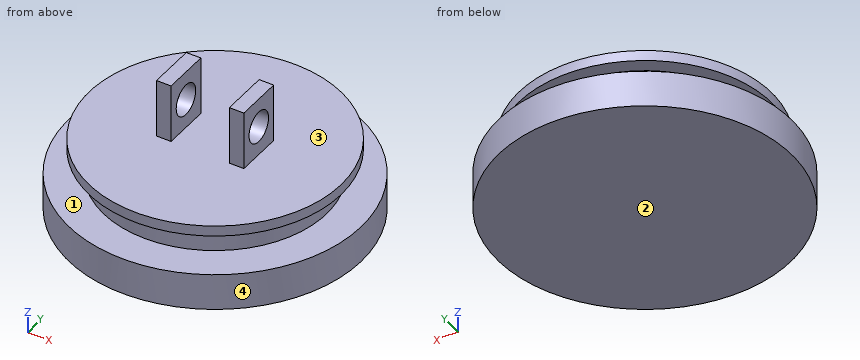
from build123d import *

# Parameters (mm, degrees)
F0_R      = 20
F1_DEPTH  = 5
F2_R      = 17.25
F3_DEPTH  = 10
F4_W      = 2
F4_H      = 3.56
F7_W      = 2
F7_H      = 6.5
F8_DEPTH  = 8
F9_R      = 2.125
F10_DEPTH = 26.001


with BuildPart() as f1:
    # F0 (on Top) → F1 (new body)
    with BuildSketch(Plane.XY):
        Circle(F0_R)
    extrude(amount=F1_DEPTH)

    # F2 (on Top) → F3 (join)
    with BuildSketch(Plane.XY):
        Circle(F2_R)
    extrude(amount=F3_DEPTH)

    # F4 (on Right) → F6 (revolve, cut)
    with BuildSketch(Plane.YZ):
        with Locations((16.25, 6.78)):
            Rectangle(F4_W, F4_H)
    revolve(axis=Axis((0, 0, 6.819869), (0, 0, 1)), mode=Mode.SUBTRACT)

    # F7 (on face) → F8 (join)
    with BuildSketch(Plane.XY.offset(10)):
        with Locations((5, 0)):
            Rectangle(F7_W, F7_H)
        with Locations((-5, 0)):
            Rectangle(F7_W, F7_H)
    extrude(amount=F8_DEPTH)

    # F9 (on face) → F10 (cut, through all)
    with BuildSketch(Plane(origin=(-6, 0, 0), x_dir=(0, -1, 0), z_dir=(-1, 0, 0))):
        with Locations((0, 14)):
            Circle(F9_R)
    extrude(amount=-F10_DEPTH, mode=Mode.SUBTRACT)


solid = f1.part
Design review of the part built by this model. Coordinates are the model's own, in mm. Face numbers are marked on the shaded views. Round coordinates to 2 decimals unless told otherwise and drop trailing zeros. Loops run counter-clockwise (first coordinate to the right, second up) from the corner with the lowest first, then second, coordinate; pieces in that order, holes last. Notation, with made-up numbers: M -29,66 L 6,66 A14 ccw 6,81 Z; hole C 25,16.5 d6. An arc over 180 degrees is marked long. Answer as a JSON object with one key per item and string values.
Item 1: We need section A-A on y = 0. Give the boundary of the cut face in (x, z) (3 decimals), and give its area (3 significant figures).
Answer sheet:
{"outline": "M -20,0 L 20,0 L 20,5 L 15.25,5 L 15.25,8.56 L 17.25,8.56 L 17.25,10 L 6,10 L 6,11.875 L 4,11.875 L 4,10 L -4,10 L -4,11.875 L -6,11.875 L -6,10 L -17.25,10 L -17.25,8.56 L -15.25,8.56 L -15.25,5 L -20,5 Z; M -6,16.125 L -4,16.125 L -4,18 L -6,18 Z; M 4,16.125 L 6,16.125 L 6,18 L 4,18 Z", "area": "373 mm^2"}
Item 2: Wall thickness on L1, parallel to Z at x = -5.15, y = 0 (3 decimals); L2, parallel to Z at x = 7, y = -13.5; L3, parallel to Y at x = 5, z = 17: over which ranges is each line inside the solid? List them lowest first. Write a range as from..to.
Answer sheet:
{"L1": "z = 0..11.875, 16.125..18", "L2": "z = 0..10", "L3": "y = -3.25..3.25"}
Item 3: The part is to be moulded in two halves that separate along Z. For the marked faces 1, 2, 3 and 4, say which applies: pulls with the +Z half, pulls with the -Z half, needs draft (parallel to the pull), parting line crosses it, or undercut.
Answer sheet:
{"face 1": "undercut", "face 2": "pulls with the -Z half", "face 3": "pulls with the +Z half", "face 4": "needs draft"}
Item 4: We need section B-B on z = 14.5. Give the boundary of the cut face in (x, y), and give its area (3 significant figures).
Answer sheet:
{"outline": "M -6,-3.25 L -4,-3.25 L -4,-2.07 L -6,-2.07 Z; M -6,2.07 L -4,2.07 L -4,3.25 L -6,3.25 Z; M 4,-3.25 L 6,-3.25 L 6,-2.07 L 4,-2.07 Z; M 4,2.07 L 6,2.07 L 6,3.25 L 4,3.25 Z", "area": "9.48 mm^2"}
Item 5: We need section C-C on y = 8.5. Give the boundary of the cut face in (x, z), and give its area (3 significant figures).
Answer sheet:
{"outline": "M -18.1,0 L 18.1,0 L 18.1,5 L 12.66,5 L 12.66,8.56 L 15.01,8.56 L 15.01,10 L -15.01,10 L -15.01,8.56 L -12.66,8.56 L -12.66,5 L -18.1,5 Z", "area": "314 mm^2"}
Item 6: Clearance check with flat-ended pins moving along their axes: P1, Ø5, axis at y = -0.5, z = 15, coming from the -X side; P2, Ø1, axis at x = -4.5, z = 13, coming from the +Y side; P3, Ø1.5, axis at x = -12.5, z = 7, coming from the +Y side. State where each tip first meets the part, or that it passes through.
Answer sheet:
{"P1": "stops at x = -6", "P2": "stops at y = 3.25", "P3": "stops at y = 9.72"}
Item 7: We need section D-D on x = 12.5. Give the boundary of the cut face in (y, z).
Answer sheet:
{"outline": "M -15.61,0 L 15.61,0 L 15.61,5 L 8.74,5 L 8.74,8.56 L 11.89,8.56 L 11.89,10 L -11.89,10 L -11.89,8.56 L -8.74,8.56 L -8.74,5 L -15.61,5 Z"}
